```python
from build123d import *

# Parameters (mm, degrees)
EXTRUDE_THIN2_DEPTH      = 1
EXTRUDE_THIN2_DEPTH_BACK = 30


with BuildPart() as part:
    # Sketch2 → Extrude-Thin2 (new, two sides: drawn at the far end of the back side and taken through both)
    with BuildSketch(Plane.XY.offset(-EXTRUDE_THIN2_DEPTH_BACK)):
        with BuildLine():
            Line((203.150311833, 38.600349755), (3.634824321, 52.423187112))
            ThreePointArc((3.634824321, 52.423187112), (-51.820262836, 4.346595446), (-3.963228019, -51.298077043))
            Line((-3.963228019, -51.298077043), (95.739880914, -58.998081537))
            ThreePointArc((95.739880914, -58.998081537), (96.149833249, -59.028112402), (96.560010162, -59.054901754))
            Line((96.560010162, -59.054901754), (196.372388742, -65.177734616))
            ThreePointArc((196.372388742, -65.177734616), (251.445709315, -16.664285771), (203.150311833, 38.600349755))
        make_face()
        with BuildLine():
            Line((203.01207914, 36.605132543), (3.496591628, 50.4279699))
            ThreePointArc((3.496591628, 50.4279699), (-49.82560756, 4.200477913), (-3.809227929, -49.304014864))
            Line((-3.809227929, -49.304014864), (95.893881004, -57.004019358))
            ThreePointArc((95.893881004, -57.004019358), (96.288065941, -57.03289519), (96.68246682, -57.058654182))
            Line((96.68246682, -57.058654182), (196.494845399, -63.181487045))
            ThreePointArc((196.494845399, -63.181487045), (249.449961335, -16.533940078), (203.01207914, 36.605132543))
        make_face(mode=Mode.SUBTRACT)
    extrude(amount=EXTRUDE_THIN2_DEPTH + EXTRUDE_THIN2_DEPTH_BACK)


solid = part.part
```
Can you work these out from the model? Positions are in its coordinate system, mm. A direction names the side the tool comes from. Give positions to 0.01 mm unless a question says otherwise; leave off trailing zeros. Order: outer loops, then holes, each group sorted by start corner. A loop starts at its lowest first (then second) coordinate and runs counter-clockwise, first axis right, second up. Notation, with made-up numbers: (-10.5, 89.25) - (31.5, 89.25) arc R15 cw to (31.5, 105.25) - close; hole circle Ø10 at (21.5, -31). An arc over 180 degrees is marked (long way). Use a Markdown table: item, result. Add a question column.
Q1. If we section it at A-A on y = -0.5: Write out the boundary of the cut face in (x, z), plus the area to 3 significant figures.
Q2. On a 3-axis mill with a long thin cutter (end or side, diameter ignored), from which of +Z, -Z, +X, -X, +Y, -Y can I reach the whole of each face in a straight line? I mean faces 1 (the flat face through (45.34, -53.1, -14.72)), 2 (the flat face through (45.19, -55.094, -14.717)). Say none if no direction works.
Q3. If we section it at C-C on x = 71: Write out the boundary of the cut face in (y, z).
Q4. Please list where these lines run through material, in increasing order: line 1 along X through (y, z) = (2, -16); line 2 along Y through (x, z) = (212.5, -25.5); line 3 along X through (y, z) = (22, -13).
Q5. I'm going to push flat-ended pins straight in: pin 1 (4 mm diameter, centred on y = -5.5, z = -11.5, fed in from -X); pin 2 (8 mm diameter, centred on y = -14, z = -17.5, fed in from +X); pin 3 (4 mm diameter, centred on y = 12.5, z = -7, fed in from -X). Where does each tip first touch, or does it pass through?
Q6. If we section it at B-B on z = -24: Write out the boundary of the cut face in (x, y).
Answers follow:
| question | item | result |
|---|---|---|
| 1 | outline | (-51.95, -30) - (-49.95, -30) - (-49.95, 1) - (-51.95, 1) - close; (247.9, -30) - (249.96, -30) - (249.96, 1) - (247.9, 1) - close |
| 1 | area | 126 mm^2 |
| 2 | face 1 | +Z, -Z |
| 2 | face 2 | +Z, -Z, -X, -Y |
| 3 | outline | (-57.09, -30) - (-55.08, -30) - (-55.08, 1) - (-57.09, 1) - close; (45.75, -30) - (47.76, -30) - (47.76, 1) - (45.75, 1) - close |
| 4 | line 1 | x = -51.94 to -49.94, 247.17 to 249.26 |
| 4 | line 2 | y = -63.64 to -61.57, 35.02 to 37.09 |
| 4 | line 3 | x = -47.33 to -45.12, 234.99 to 237.76 |
| 5 | pin 1 | stops at x = -51.8 |
| 5 | pin 2 | stops at x = 251.56 |
| 5 | pin 3 | stops at x = -51 |
| 6 | outline | (-3.96, -51.3) - (95.74, -59) arc R52 ccw to (96.56, -59.05) - (196.37, -65.18) arc R52 ccw to (203.15, 38.6) - (3.63, 52.42) arc R52 ccw to start; hole (-3.81, -49.3) - (95.89, -57) arc R50 ccw to (96.68, -57.06) - (196.49, -63.18) arc R50 ccw to (203.01, 36.61) - (3.5, 50.43) arc R50 ccw to start |
